```python
from build123d import *

# Parameters (mm, degrees)
SKETCH_4_W          = 16.2
SKETCH_4_H          = 14.2
SKETCH_4_R          = 1.75
SKETCH_4_R_2        = 0.9
EXTRUDE_1_DEPTH     = 2
SKETCH_4_8_W        = 16.2
SKETCH_4_8_H        = 14.2
SKETCH_4_8_W_2      = 12.2
SKETCH_4_8_H_2      = 10.2
EXTRUDE_2_DEPTH     = 3
SKETCH_5_W          = 3.55
SKETCH_5_H          = 14.2
EXTRUDE_3_DEPTH     = 2
SKETCH_6_R          = 1
CUT_EXTRUDE_1_DEPTH = 14.968983499


with BuildPart() as part:
    # Sketch 4 → Extrude 1 (new body)
    with BuildSketch(Plane(origin=(0, 0, 0), x_dir=(1, 0, 0), z_dir=(0, 1, 0))):
        Rectangle(SKETCH_4_W, SKETCH_4_H)
        with Locations(Location((0, 0, 0), (0, 0, 270))):
            Circle(SKETCH_4_R, mode=Mode.SUBTRACT)
        with Locations(Location((-4.5, 0, 0), (0, 0, 270))):
            Circle(SKETCH_4_R_2, mode=Mode.SUBTRACT)
        with Locations(Location((4.5, 0, 0), (0, 0, 270))):
            Circle(SKETCH_4_R_2, mode=Mode.SUBTRACT)
    extrude(amount=EXTRUDE_1_DEPTH)

    # Sketch 4_8 → Extrude 2 (add)
    with BuildSketch(Plane(origin=(0, 0, 0), x_dir=(1, 0, 0), z_dir=(0, 1, 0))):
        Rectangle(SKETCH_4_8_W, SKETCH_4_8_H)
        Rectangle(SKETCH_4_8_W_2, SKETCH_4_8_H_2, mode=Mode.SUBTRACT)
    extrude(amount=-EXTRUDE_2_DEPTH)

    # Sketch 5 → Extrude 3 (add)
    with BuildSketch(Plane(origin=(0, 2, 0), x_dir=(1, 0, 0), z_dir=(0, 1, 0))):
        with Locations((9.875, 0)):
            Rectangle(SKETCH_5_W, SKETCH_5_H)
        with Locations((-9.875, 0)):
            Rectangle(SKETCH_5_W, SKETCH_5_H)
    extrude(amount=-EXTRUDE_3_DEPTH)

    # Sketch 6 → Cut-Extrude 1 (cut, through all)
    with BuildSketch(Plane(origin=(0, 0, 0), x_dir=(-1, 0, 0), z_dir=(0, -1, 0))):
        with Locations(Location((-9.875, 0, 0), (0, 0, 90))):
            Circle(SKETCH_6_R)
        with Locations(Location((9.875, 0, 0), (0, 0, 90))):
            Circle(SKETCH_6_R)
    extrude(amount=-CUT_EXTRUDE_1_DEPTH, mode=Mode.SUBTRACT)


solid = part.part
```
Check sheet for the modelled part. Datum: model origin and axes. Units: mm. A direction names the side the tool comes from. Round coordinates to 2 decimals unless told otherwise and drop trailing zeros. Loops run counter-clockwise (first coordinate to the right, second up) from the corner with the lowest first, then second, coordinate; pieces in that order, holes last. Notation, with made-up numbers: M 71,-14 L 80,-14 A29 cw 80,14 Z; hole C -11,-6.5 d4. An arc over 180 degrees is marked long. Answer as a JSON object with one key per item and string values.
1. Section check A-A (z = 0). State how many separate pieces and enclosed holes the cut face has, plus the area to 3 significant figures.
Reply:
{"separate pieces": "6", "enclosed holes": "0", "area": "36.4 mm²"}
2. Scan lines: line 1 (X direction, y = 0.45, z = 0) (3 decimals); line 2 (Z direction, x = -5.25, y = -2.8); line 3 (X direction, y = -0.85, z = 2.25). Record each from-to range of solid material in increasing order.
Reply:
{"line 1": "x = -11.65 to -10.875, -8.875 to -5.4, -3.6 to -1.75, 1.75 to 3.6, 5.4 to 8.875, 10.875 to 11.65", "line 2": "z = -7.1 to -5.1, 5.1 to 7.1", "line 3": "x = -8.1 to -6.1, 6.1 to 8.1"}
3. Section check D-D (z = 2.5). Record the boundary of the cut face in (x, y).
Reply:
{"outline": "M -11.65,0 L -8.1,0 L -8.1,-3 L -6.1,-3 L -6.1,0 L 6.1,0 L 6.1,-3 L 8.1,-3 L 8.1,0 L 11.65,0 L 11.65,2 L -11.65,2 Z"}
4. Section check B-B (x = -4.5). Record the boundary of the cut face in (y, z), plus the area to 3 significant figures.
Reply:
{"outline": "M -3,-7.1 L 2,-7.1 L 2,-0.9 L 0,-0.9 L 0,-5.1 L -3,-5.1 Z; M -3,5.1 L 0,5.1 L 0,0.9 L 2,0.9 L 2,7.1 L -3,7.1 Z", "area": "36.8 mm²"}
5. Gauge pin test, flat ends, axial feed: P1, Ø2.5, axis at y = -2, z = -1.5, coming from the +X side; P2, Ø3, axis at x = -10.5, z = 1, coming from the -Y side; P3, Ø2.5, axis at x = 9.875, z = 0, coming from the +Y side; P4, Ø0.9, axis at y = -2, z = 1, coming from the -X side. Record the tip position at first contact, or that the pin passes through.
Reply:
{"P1": "stops at x = 8.1", "P2": "stops at y = 0", "P3": "stops at y = 2", "P4": "stops at x = -8.1"}
6. Mould release check, pull along X, two halves, no side actions. Record for faces 1 (the flat face through (0, 0, -2)), 2 (the flat face through (0, -1, -5.1)), 3 (the flat face through (0, 0, -7.1)), 4 (the flat face through (11.65, 1, 0)): pulls with the +X half, pulls with the -X half, needs draft (parallel to the pull), parting line crosses it, or undercut.
Reply:
{"face 1": "undercut", "face 2": "undercut", "face 3": "needs draft", "face 4": "pulls with the +X half"}
7. Access from +Z, -Z, +X, -X, +Y, -Y to the whole of each face (thin tool, end or side, straight path). Record for faces 5 (the cylindrical face through (-5.379, 0.986, -0.195)), 6 (the flat face through (6.1, -1, 0)), 7 (the flat face through (8.1, -1, 0)), 8 (the flat face through (-11.1, 0, -0.1)).
Reply:
{"face 5": "+Y, -Y", "face 6": "-Y", "face 7": "+Z, -Z, +X, -Y", "face 8": "+Z, -Z, -X, -Y"}
8. Section check C-C (y = -2.1). Record the boundary of the cut face in (x, z).
Reply:
{"outline": "M -8.1,-7.1 L 8.1,-7.1 L 8.1,7.1 L -8.1,7.1 Z; hole M -6.1,-5.1 L 6.1,-5.1 L 6.1,5.1 L -6.1,5.1 Z"}
